Geometry check sheet. Reference: the model listing, model coordinates, mm. A direction names the side the tool comes from. Round coordinates to 2 decimals unless told otherwise and drop trailing zeros. Loops run counter-clockwise (first coordinate to the right, second up) from the corner with the lowest first, then second, coordinate; pieces in that order, holes last. Notation, with made-up numbers: (-4.5, 83) -> (50.5, 83) arc R22 ccw to (50.5, 100) -> close; hole circle Ø7 at (16, 27). An arc over 180 degrees is marked (long way). Use a Markdown table: item, result. Add a question column.
Q1. Sectioned sample at B-B, the plane z = 3.05. Enter the section's corners in (x, y), then the cut area to 3 significant figures.
Q2. Sectioned sample at C-C, the plane x = 45.5. Enter the section's corners in (y, z), then the cut area to 3 significant figures.
Q3. Sectioned sample at A-A, the plane y = 26.5. Enter the section's corners in (x, z), then the cut area to 3 significant figures.
Q4. Gauge pin test, flat end, axial feed: P1, Ø2, axis at x = 251.5, z = 2, coming from the -Y side. Record the tip position at first contact, or that the pin passes through.
Q5. Set-up check for faces 1 (the face through (-202.34, -7.85, 2.03)), 2 (the face through (15, 32, 0)): record each of +Z, -Z, +X, -X, +Y, -Y from which the full face is reachable in a straight line by a thin tool's end or side.
Q6. Sectioned sample at D-D, the plane y = -36.5. Enter the section's corners in (x, z).
Q7. Material ranges on L1, parallel to X at y = -15, z = 2.6; L2, parallel to X at y = -18.5, z = 1.5; L3, parallel to Y at x = -36, z = 2.1, recorded low to high.
```python
from build123d import *

# Parameters (mm, degrees)
F1_DEPTH = 4
F2_R     = 54.0232948569
F3_R     = 62.809614709
F4_W     = 34.3843554476
F4_H     = 20.342006709
F5_DEPTH = 4
F7_R     = 20


with BuildPart() as f1:
    # F0 (on Top) → F1 (new body)
    with BuildSketch(Plane.XY):
        with BuildLine():
            ThreePointArc((-214.4679278135, 0), (8.6127225609, 31.0011100466), (231.6933729353, 0))
            Line((231.6933729353, 0), (231.6933729353, -24.0185298026))
            Line((231.6933729353, -24.0185298026), (266.0777283828, -24.0185298026))
            Line((266.0777283828, -24.0185298026), (266.0777283828, 0))
            ThreePointArc((266.0777283828, 0), (16.0777283828, 58.0256148842), (-233.9222716172, 0))
            Line((-233.9222716172, 0), (-233.9222716172, -50))
            ThreePointArc((-233.9222716172, -50), (-224.3045684517, -45.7747103429), (-214.4679278135, -49.461685773))
            Line((-214.4679278135, -49.461685773), (-214.4679278135, 0))
        make_face()
    extrude(amount=F1_DEPTH)

    # F2
    f2_edges = [f1.edges().sort_by_distance(p)[0] for p in [
        (-214.467928, 0, 2),
    ]]
    fillet(f2_edges, radius=F2_R)

    # F3
    f3_edges = [f1.edges().sort_by_distance(p)[0] for p in [
        (-233.922272, 0, 2),
    ]]
    fillet(f3_edges, radius=F3_R)

    # F7
    f7_edges = [f1.edges().sort_by_distance(p)[0] for p in [
        (266.077728, 0, 2),
        (231.693373, 0, 2),
    ]]
    fillet(f7_edges, radius=F7_R)


with BuildPart() as f5:
    # F4 (on face) → F5 (new body)
    with BuildSketch(Plane.XY.offset(4)):
        with Locations((248.885550659, -10.1710033545)):
            Rectangle(F4_W, F4_H)
    extrude(amount=F5_DEPTH)


solid = f1.part
```
Values:
| question | item | result |
|---|---|---|
| 1 | outline | (-233.92, -50) arc R13.94 cw to (-214.47, -49.46) -> (-214.47, -41.96) arc R54.02 cw to (-172.4, 10.73) arc R818.13 cw to (216.78, 4.07) arc R20 cw to (231.69, -15.27) -> (231.69, -24.02) -> (266.08, -24.02) -> (266.08, -12.62) arc R20 ccw to (254.48, 5.53) arc R567.57 ccw to (-194.41, 17.55) arc R62.81 ccw to (-233.92, -40.78) -> close |
| 1 | area | 12,100 mm^2 |
| 2 | outline | (30.17, 0) -> (57.26, 0) -> (57.26, 4) -> (30.17, 4) -> close |
| 2 | area | 108 mm^2 |
| 3 | outline | (-170.45, 0) -> (-77.09, 0) -> (-77.09, 4) -> (-170.45, 4) -> close; (94.31, 0) -> (202.6, 0) -> (202.6, 4) -> (94.31, 4) -> close |
| 3 | area | 807 mm^2 |
| 4 | P1 | y = -24.02 |
| 5 | face 1 | +Z, -Z, -Y |
| 5 | face 2 | -Z, +X, -X, +Y, -Y |
| 6 | outline | (-233.78, 0) -> (-214.19, 0) -> (-214.19, 4) -> (-233.78, 4) -> close |
| 7 | L1 | -228.39 to -207.26, 231.69 to 266.08 |
| 7 | L2 | -229.84 to -209.11, 231.69 to 266.08 |
| 7 | L3 | 29.78 to 55.63 |
